Here's how the part is built. I have some questions about the finished solid (model axes, mm). Coordinates: 2 decimals unless noted, no trailing zeros. Write each loop counter-clockwise with the first axis right and the second up, starting at its lowest first coordinate (ties: lowest second). Pieces come first, ordered by that corner, then holes.
Item 1: If we mould it in two halves opening along X, with no side actions, what happens to faces 1 (the face through (-20.79, -20.18, 2.71)), 2 (the face through (-34.15, -1, 3)), 3 (the face through (0, 1, 0))? For each: pulls with the +X half, pulls with the -X half, needs draft (parallel to the pull), parting line crosses it, or undercut.
Item 2: I want a section at A-A (y = -19). Please give me the cut outline in (x, z), and give its area (3 significant figures).
Item 3: I want a section at B-B (z = 2.25). Count the separate pieces of the cut face and the enclosed holes in it, and give its area (3 significant figures).
Item 4: Please list where these lines run through material, in increasing order: line 1 (X direction, y = 19, z = 3.15); line 2 (Y direction, x = 18, z = 1.75); line 3 (X direction, y = 36.5, z = 6.25).
Item 5: I want a section at C-C (x = -19.5). Please give me the cut outline in (y, z), and give its area (3 significant figures).
Item 6: I want a section at D-D (y = 34.8). Please give me the cut outline in (x, z).
Autodesk Fusion 360 part; units mm, degrees
sketch "Sketch1" plane through (0, 0, 0) normal (0, 0, 1) x (1, 0, 0)
  line L0 (-34.15, 48.95) -> (34.15, 48.95)
  line L1 (34.15, 48.95) -> (34.15, -48.95)
  line L2 (34.15, -48.95) -> (-34.15, -48.95)
  line L3 (-34.15, -48.95) -> (-34.15, 48.95)
  line L4 (-34.15, 48.95) -> (34.15, -48.95) construction
  line L5 (34.15, 48.95) -> (-34.15, -48.95) construction
  line L6 (19.5, 19) -> (-19.5, 19) construction
  line L7 (-19.5, 19) -> (-19.5, -19) construction
  line L8 (-19.5, -19) -> (19.5, -19) construction
  line L9 (19.5, -19) -> (19.5, 19) construction
  line L10 (19.5, 19) -> (-19.5, -19) construction
  line L11 (-19.5, 19) -> (19.5, -19) construction
  circle A0 centre (-19.5, 19) radius 1.75
  circle A1 centre (19.5, 19) radius 1.75
  circle A2 centre (19.5, -19) radius 1.75
  circle A3 centre (-19.5, -19) radius 1.75
  line L12 (0, 1.75) -> (0, 22.5)
  line L13 (1.75, 0) -> (22.5, 0)
  line L14 (20, 34.8) -> (-20, 34.8) construction
  line L15 (-20, 34.8) -> (-20, -34.8) construction
  line L16 (-20, -34.8) -> (20, -34.8) construction
  line L17 (20, -34.8) -> (20, 34.8) construction
  line L18 (20, 34.8) -> (-20, -34.8) construction
  line L19 (-20, 34.8) -> (20, -34.8) construction
  circle A4 centre (-20, 34.8) radius 4.25
  circle A5 centre (20, 34.8) radius 4.25
  circle A6 centre (20, -34.8) radius 4.25
  circle A7 centre (-20, -34.8) radius 4.25
  dimension "d3" = 39
  dimension "d4" = 38
  dimension "d5" = 3.5
  dimension "d10" = 40
  dimension "d11" = 8.5
  dimension "d12" = 15.8
  dimension "d13" = 14.15
  dimension "d16" = 68.3
extrude "Extrude2" add sketch "Sketch1" along normal blind 7
sketch "Sketch2" plane through (0, 0, 7) normal (0, 0, 1) x (-1, 0, 0)
  circle A0 centre (-19.5, 19) radius 1.75
  circle A1 centre (19.5, 19) radius 1.75
  circle A2 centre (19.5, -19) radius 1.75
  circle A3 centre (-19.5, -19) radius 1.75
  circle A4 centre (20, -34.8) radius 4.25
  circle A5 centre (-20, -34.8) radius 4.25
  circle A6 centre (-20, 34.8) radius 4.25
  circle A7 centre (20, 34.8) radius 4.25
  line L0 (34.15, 48.95) -> (-34.15, 48.95)
  line L1 (-34.15, 48.95) -> (-34.15, -48.95)
  line L2 (-34.15, -48.95) -> (34.15, -48.95)
  line L3 (34.15, -48.95) -> (34.15, 48.95)
  circle A8 centre (19.5, 19) radius 3
  circle A9 centre (-19.5, 19) radius 3
  circle A10 centre (-19.5, -19) radius 3
  circle A11 centre (19.5, -19) radius 3
  dimension "d17" = 6
hole "Hole1" at (19.5, 19, 7) direction (0, 0, -1) diameter 3 depth 10 tip angle 118 countersink diameter 6.5 countersink angle 90
hole "Hole2" at (-19.5, 19, 7) direction (0, 0, -1) diameter 3 depth 16 tip angle 118 countersink diameter 6.5 countersink angle 90
hole "Hole3" at (-19.5, -19, 7) direction (0, 0, -1) diameter 3 depth 16 tip angle 118 countersink diameter 6.5 countersink angle 90
hole "Hole4" at (19.5, -19, 7) direction (0, 0, -1) diameter 3 depth 16 tip angle 118 countersink diameter 6.5 countersink angle 90
equation "d12 = 10 mm + ( 3.3 / 2 ) * 1 mm + ( 8.3 / 2 ) * 1 mm"
equation "d13 = 10 mm + ( 8.3 / 2 ) * 1 mm"
equation "d16 = 40 mm + 8.3 mm + 20 mm"
Answer:
1. face 1: undercut
1. face 2: pulls with the -X half
1. face 3: needs draft
2. outline: (-34.15, 0) - (-21.25, 0) - (-21.25, 5.5) - (-22.75, 7) - (-34.15, 7) - close; (-17.75, 0) - (17.75, 0) - (17.75, 5.5) - (16.25, 7) - (-16.25, 7) - (-17.75, 5.5) - close; (21.25, 0) - (34.15, 0) - (34.15, 7) - (22.75, 7) - (21.25, 5.5) - close
2. area: 425 mm2
3. separate pieces: 1
3. enclosed holes: 8
3. area: 6,420 mm2
4. line 1: x = -34.15 to -21.25, -17.75 to 17.75, 21.25 to 34.15
4. line 2: y = -48.95 to -38.55, -31.05 to -19.9, -18.1 to 18.1, 19.9 to 31.05, 38.55 to 48.95
4. line 3: x = -34.15 to -23.9, -16.1 to 16.1, 23.9 to 34.15
5. outline: (-48.95, 0) - (-39.02, 0) - (-39.02, 7) - (-48.95, 7) - close; (-30.58, 0) - (-20.75, 0) - (-20.75, 5.5) - (-22.25, 7) - (-30.58, 7) - close; (-17.25, 0) - (17.25, 0) - (17.25, 5.5) - (15.75, 7) - (-15.75, 7) - (-17.25, 5.5) - close; (20.75, 0) - (30.58, 0) - (30.58, 7) - (22.25, 7) - (20.75, 5.5) - close; (39.02, 0) - (48.95, 0) - (48.95, 7) - (39.02, 7) - close
5. area: 514 mm2
6. outline: (-34.15, 0) - (-24.25, 0) - (-24.25, 7) - (-34.15, 7) - close; (-15.75, 0) - (15.75, 0) - (15.75, 7) - (-15.75, 7) - close; (24.25, 0) - (34.15, 0) - (34.15, 7) - (24.25, 7) - close
